from build123d import *

# Parameters (mm, degrees)
SKETCH1_W           = 25.4
SKETCH1_H           = 239.7125
BOSS_EXTRUDE1_DEPTH = 1.5875
CUT_EXTRUDE1_DEPTH  = 1.5875


with BuildPart() as part:
    # Sketch1 → Boss-Extrude1 (new body)
    with BuildSketch(Plane(origin=(0, 0, 0), x_dir=(1, 0, 0), z_dir=(0, 1, 0))):
        Rectangle(SKETCH1_W, SKETCH1_H)
    extrude(amount=BOSS_EXTRUDE1_DEPTH)

    # Sketch2 → Cut-Extrude1 (cut)
    with BuildSketch(Plane(origin=(0, 1.5875, 0), x_dir=(1, 0, 0), z_dir=(0, 1, 0))):
        with BuildLine():
            Line((-4.168311679, -107.15625), (6.0325, -107.15625))
            ThreePointArc((6.0325, -107.15625), (7.155032015, -106.691282015), (7.62, -105.56875))
            Line((7.62, -105.56875), (7.62, -74.018760533))
            ThreePointArc((7.62, -74.018760533), (6.279706302, -72.450626198), (4.521990181, -73.530379191))
            Line((4.521990181, -73.530379191), (-5.678821499, -105.080368658))
            ThreePointArc((-5.678821499, -105.080368658), (-5.451951355, -106.50278717), (-4.168311679, -107.15625))
        make_face()
        with BuildLine():
            Line((-4.7625, 114.77625), (5.407956322, 114.77625))
            ThreePointArc((5.407956322, 114.77625), (6.691595997, 114.12278717), (6.918466141, 112.700368658))
            Line((6.918466141, 112.700368658), (-3.251990181, 81.244264977))
            ThreePointArc((-3.251990181, 81.244264977), (-5.009706302, 80.164511984), (-6.35, 81.732646319))
            Line((-6.35, 81.732646319), (-6.35, 113.18875))
            ThreePointArc((-6.35, 113.18875), (-5.885032015, 114.311282015), (-4.7625, 114.77625))
        make_face()
        with BuildLine():
            Line((7.62, 88.287239467), (7.62, 61.81725))
            ThreePointArc((7.62, 61.81725), (7.155032015, 60.694717985), (6.0325, 60.22975))
            Line((6.0325, 60.22975), (-2.525834956, 60.22975))
            ThreePointArc((-2.525834956, 60.22975), (-3.809474631, 60.88321283), (-4.036344775, 62.305631342))
            Line((-4.036344775, 62.305631342), (4.521990181, 88.775620809))
            ThreePointArc((4.521990181, 88.775620809), (6.279706302, 89.855373802), (7.62, 88.287239467))
        make_face()
        with BuildLine():
            Line((-3.251990181, -81.061735023), (5.132272704, -55.130131342))
            ThreePointArc((5.132272704, -55.130131342), (4.90540256, -53.70771283), (3.621762885, -53.05425))
            Line((3.621762885, -53.05425), (-4.7625, -53.05425))
            ThreePointArc((-4.7625, -53.05425), (-5.885032015, -53.519217985), (-6.35, -54.64175))
            Line((-6.35, -54.64175), (-6.35, -80.573353681))
            ThreePointArc((-6.35, -80.573353681), (-5.009706302, -82.141488016), (-3.251990181, -81.061735023))
        make_face()
        with BuildLine():
            Line((-3.251990181, -26.959735023), (5.132272704, -1.028131342))
            ThreePointArc((5.132272704, -1.028131342), (4.90540256, 0.39428717), (3.621762885, 1.04775))
            Line((3.621762885, 1.04775), (-4.7625, 1.04775))
            ThreePointArc((-4.7625, 1.04775), (-5.885032015, 0.582782015), (-6.35, -0.53975))
            Line((-6.35, -0.53975), (-6.35, -26.471353681))
            ThreePointArc((-6.35, -26.471353681), (-5.009706302, -28.039488016), (-3.251990181, -26.959735023))
        make_face()
        with BuildLine():
            Line((-4.036344775, -45.898368658), (4.521990181, -19.428379191))
            ThreePointArc((4.521990181, -19.428379191), (6.279706302, -18.348626198), (7.62, -19.916760533))
            Line((7.62, -19.916760533), (7.62, -46.38675))
            ThreePointArc((7.62, -46.38675), (7.155032015, -47.509282015), (6.0325, -47.97425))
            Line((6.0325, -47.97425), (-2.525834956, -47.97425))
            ThreePointArc((-2.525834956, -47.97425), (-3.809474631, -47.32078717), (-4.036344775, -45.898368658))
        make_face()
        with BuildLine():
            Line((-3.251990181, 27.142264977), (5.132272704, 53.073868658))
            ThreePointArc((5.132272704, 53.073868658), (4.90540256, 54.49628717), (3.621762885, 55.14975))
            Line((3.621762885, 55.14975), (-4.7625, 55.14975))
            ThreePointArc((-4.7625, 55.14975), (-5.885032015, 54.684782015), (-6.35, 53.56225))
            Line((-6.35, 53.56225), (-6.35, 27.630646319))
            ThreePointArc((-6.35, 27.630646319), (-5.009706302, 26.062511984), (-3.251990181, 27.142264977))
        make_face()
        with BuildLine():
            Line((-4.707523276, 6.12775), (4.521990181, 34.673620809))
            ThreePointArc((4.521990181, 34.673620809), (6.279706302, 35.753373802), (7.62, 34.185239467))
            Line((7.62, 34.185239467), (7.62, 7.71525))
            ThreePointArc((7.62, 7.71525), (7.155032015, 6.592717985), (6.0325, 6.12775))
            Line((6.0325, 6.12775), (-4.707523276, 6.12775))
        make_face()
    extrude(amount=-CUT_EXTRUDE1_DEPTH, mode=Mode.SUBTRACT)


solid = part.part
Input: part model. Units: mm. Frame: model coordinates. A direction names the side the tool comes from. Coordinates: 2 decimals unless noted, no trailing zeros. Order: outer loops, then holes, each group sorted by start corner. A loop starts at its lowest first (then second) coordinate and runs counter-clockwise, first axis right, second up. Notation, with made-up numbers: M 60,24 L 73,24 A13 ccw 73,43 Z; hole C 55.5,65.5 d3. An arc over 180 degrees is marked long. One line per question, with ' | ' between items.
Item 1: Section A-A (z = 23). Output: boundary loops of the cut face in (x, y).
Geometry results:
outline: M -12.7,0 L -6.35,0 L -6.35,1.59 L -12.7,1.59 Z; M -1.97,0 L 3.37,0 L 3.37,1.59 L -1.97,1.59 Z; M 7.62,0 L 12.7,0 L 12.7,1.59 L 7.62,1.59 Z
Item 2: Reachability of faces 1 (the flat face through (0, 1.588, -2)), 2 (the flat face through (0.88, 0.8, 14.18)) from +Z, -Z, +X, -X, +Y, -Y: full face, straight path, thin tool, end or side. Return the list, or none.
Geometry results:
face 1: +Z, -Z, +X, -X, +Y | face 2: +Y, -Y
Item 3: Ray query, line 1 along X through (y, z) = (0.9, -53.5); line 2 along X through (y, z) = (0.25, -34); line 3 along X through (y, z) = (0.55, 105). Return the intervals inside material, ascending.
Geometry results:
line 1: x = -12.7 to -6.35, 5.21 to 12.7 | line 2: x = -12.7 to -6.35, -1.03 to 4.3, 7.62 to 12.7 | line 3: x = -12.7 to -5.65, 7.62 to 12.7
Item 4: Pin query (flat end, axial travel): pin 1 (5 mm diameter, centred on x = -4, z = 89.5, fed in from -Y). Return the tip coordinate at first contact, or that it passes through.
Geometry results:
pin 1: stops at y = 0
Item 5: Draft query along X for faces 3 (the flat face through (0.183, 0.805, -75.355)), 4 (the flat face through (0, 0, -2)). Return one class per face: released by +X, released by -X, zero draft, split by the parting line, or undercut.
Geometry results:
face 3: undercut | face 4: zero draft
Item 6: Section B-B (y = 0.9). Give the number of separate pieces and of enclosed holes in the cut face, then the cut area to 3 significant figures.
Geometry results:
separate pieces: 1 | enclosed holes: 8 | area: 4,210 mm^2
